Can you work these out from the model? Positions are in its coordinate system, mm. A direction names the side the tool comes from. Coordinates: 2 decimals unless noted, no trailing zeros. Loops run counter-clockwise (first coordinate to the right, second up) from the corner with the lowest first, then second, coordinate; pieces in that order, holes last. Notation, with made-up numbers: M 47.25,8.5 L 56.25,8.5 A23 cw 56.25,27.5 Z; hole C 11.5,-3.5 d6. An arc over 180 degrees is marked long. Return JSON: item names as keys, results as strings. Group by question number.
```python
from build123d import *

# Parameters (mm, degrees)
F0_W     = 501.65
F0_H     = 82.55
F0_W_2   = 19.05
F0_H_2   = 19.05
F1_DEPTH = 12.7
F2_DEPTH = 25.4
F3_DEPTH = 12.7


with BuildPart() as f1:
    # F0 (on Top) → F1 (new body)
    with BuildSketch(Plane.XY):
        with Locations((-50.692200847, -66.2992455751)):
            Rectangle(F0_W, F0_H)
        with Locations((-311.042200847, -66.2992455751)):
            Rectangle(F0_W_2, F0_H)
        with Locations((-50.692200847, -15.4992455751)):
            Rectangle(F0_W, F0_H_2)
        with Locations((209.657799153, -66.2992455751)):
            Rectangle(F0_W_2, F0_H)
    extrude(amount=F1_DEPTH)

    # F0 (on Top) → F2 (join)
    with BuildSketch(Plane.XY):
        with Locations((-50.692200847, -66.2992455751)):
            Rectangle(F0_W, F0_H)
        with Locations((-311.042200847, -66.2992455751)):
            Rectangle(F0_W_2, F0_H)
        with Locations((209.657799153, -66.2992455751)):
            Rectangle(F0_W_2, F0_H)
    extrude(amount=F2_DEPTH)

    # F0 (on Top) → F3 (cut)
    with BuildSketch(Plane.XY):
        with Locations((-311.042200847, -66.2992455751)):
            Rectangle(F0_W_2, F0_H)
        with Locations((209.657799153, -66.2992455751)):
            Rectangle(F0_W_2, F0_H)
    extrude(amount=F3_DEPTH, mode=Mode.SUBTRACT)


solid = f1.part
```
1) If I drill on line 1 (Y direction, x = 111.5, z = 20.5); line 2 (X direction, y = -59.5, z = 1.5); line 3 (Z direction, x = 56, y = -16), over which ranges is the centre line in solid material (lowest first)? Write a range as from..to.
2) For pin 1 (8 mm diameter, centred on x = -250, y = -90, fed in from -Z); pin 2 (4 mm diameter, centred on x = 66, z = 20.5, fed in from +Y); pin 3 (15 mm diameter, centred on x = 210.5, y = -81, fed in from -Z); pin 4 (4 mm diameter, centred on y = -77, z = 4.5, fed in from +X), each with a flat end and sliding along its axis, tell me the tip position at first contact or that it passes through.
3) Suppose I cut it at C-C, the plane z = 21. List the corners of the cut face in (x, y) for me, then the cut area to 3 significant figures.
4) Suppose I cut it at A-A, the plane y = -43. List the corners of the cut face in (x, z) for me, then the cut area to 3 significant figures.
5) Suppose I cut it at D-D, the plane y = -13.5. List the corners of the cut face in (x, z) for me, then the cut area to 3 significant figures.
6) For faces 1 (the face through (210, -66, 12.7)), 2 (the face through (-54, -25.024, 19)), 3 (the face through (-54, -66, 25.4)), 4 (the face through (-301.517, -57, 6)), which set-ups out of +Z, -Z, +X, -X, +Y, -Y let a thin tool reach every point of the face, with its end or its side?
7) Suppose I cut it at B-B, the plane x = -55.5. List the corners of the cut face in (y, z) for me.
Returned:
{
 "1": {"line 1": "y = -107.57..-25.02", "line 2": "x = -301.52..200.13", "line 3": "z = 0..12.7"},
 "2": {"pin 1": "stops at z = 0", "pin 2": "stops at y = -25.02", "pin 3": "stops at z = 12.7", "pin 4": "stops at x = 200.13"},
 "3": {"outline": "M -320.57,-107.57 L 219.18,-107.57 L 219.18,-25.02 L -320.57,-25.02 Z", "area": "44,600 mm²"},
 "4": {"outline": "M -320.57,12.7 L -301.52,12.7 L -301.52,0 L 200.13,0 L 200.13,12.7 L 219.18,12.7 L 219.18,25.4 L -320.57,25.4 Z", "area": "13,200 mm²"},
 "5": {"outline": "M -301.52,0 L 200.13,0 L 200.13,12.7 L -301.52,12.7 Z", "area": "6,370 mm²"},
 "6": {"face 1": "-Z, +X, +Y, -Y", "face 2": "+Z, +X, -X, +Y", "face 3": "+Z, +X, -X, +Y, -Y", "face 4": "-Z, -X, +Y, -Y"},
 "7": {"outline": "M -107.57,0 L -5.97,0 L -5.97,12.7 L -25.02,12.7 L -25.02,25.4 L -107.57,25.4 Z"}
}
